Can you work these out from the model? Positions are in its coordinate system, mm. A direction names the side the tool comes from. Give positions to 0.01 mm unless a question says otherwise; leave off trailing zeros. Write each loop counter-clockwise with the first axis right and the second up, starting at its lowest first coordinate (ties: lowest second). Pieces come first, ordered by that corner, then holes. Notation, with made-up numbers: M 86,29.5 L 130,29.5 A10 ccw 130,35.5 Z; hole C -27,-25.5 d4. An arc over 180 degrees is marked long. Use CSV: the item, a comma, the result in double quotes. Start each with the question number.
from build123d import *

# Parameters (mm, degrees)
SKETCH_1_R               = 8
EXTRUDE_1_DEPTH          = 19.5
SKETCH_2_R               = 21
EXTRUDE_2_DEPTH          = 4
SKETCH_3_R               = 1.525
CUT_EXTRUDE_1_DEPTH      = 4
SKETCH_5_W               = 16
SKETCH_5_H               = 19.5
EXTRUDE_3_DEPTH          = 8
SKETCH_8_R               = 5
EXTRUDE_4_DEPTH          = 10
HOLE_WIZARD_G1_8_1_D     = 8.8
HOLE_WIZARD_G1_8_1_DEPTH = 11
HOLE_WIZARD_G1_8_1_TIP   = 2.643786724
CUT_EXTRUDE_4_REACH      = 35.5
SKETCH_9_R               = 2.025
FILLET_1_R               = 2
CHAMFER_1_SIZE           = 0.5


with BuildPart() as part:
    # 草图1 → 凸台-拉伸1 (new body)
    with BuildSketch(Plane(origin=(0, 0, 0), x_dir=(1, 0, 0), z_dir=(0, 1, 0))):
        Circle(SKETCH_1_R)
    extrude(amount=EXTRUDE_1_DEPTH)

    # 草图2 → 凸台-拉伸2 (add)
    with BuildSketch(Plane(origin=(0, 19.5, 0), x_dir=(1, 0, 0), z_dir=(0, 1, 0))):
        Circle(SKETCH_2_R)
    extrude(amount=EXTRUDE_2_DEPTH)

    # 草图3 → 切除-拉伸1 (cut)
    with BuildSketch(Plane.XZ.offset(-19.5)):
        with Locations((0, -13.5)):
            Circle(SKETCH_3_R)
        with Locations((-11.691342951, -6.75)):
            Circle(SKETCH_3_R)
        with Locations((-11.691342951, 6.75)):
            Circle(SKETCH_3_R)
        with Locations((0, 13.5)):
            Circle(SKETCH_3_R)
        with Locations((11.691342951, 6.75)):
            Circle(SKETCH_3_R)
        with Locations((11.691342951, -6.75)):
            Circle(SKETCH_3_R)
    extrude(amount=-CUT_EXTRUDE_1_DEPTH, mode=Mode.SUBTRACT)

    # 草图5 → 凸台-拉伸3 (add)
    with BuildSketch(Plane.XY):
        with Locations((0, 9.75)):
            Rectangle(SKETCH_5_W, SKETCH_5_H)
    extrude(amount=EXTRUDE_3_DEPTH)

    # 草图8 → 凸台-拉伸4 (add)
    with BuildSketch(Plane.XZ):
        Circle(SKETCH_8_R)
    extrude(amount=EXTRUDE_4_DEPTH)

    # G1/8 螺纹孔1
    with Locations(Plane(origin=(0, 9.75, 8), x_dir=(1, 0, 0), z_dir=(0, 0, 1))):
        with Locations((0, 0)):
            Hole(HOLE_WIZARD_G1_8_1_D / 2, depth=HOLE_WIZARD_G1_8_1_DEPTH)
            with Locations((0, 0, -(HOLE_WIZARD_G1_8_1_DEPTH + HOLE_WIZARD_G1_8_1_TIP / 2))):  # 118° drill point
                Cone(0, HOLE_WIZARD_G1_8_1_D / 2, HOLE_WIZARD_G1_8_1_TIP, mode=Mode.SUBTRACT)

    # 草图9 → 切除-拉伸4 (cut, up to next)
    with BuildSketch(Plane.XZ.offset(10), mode=Mode.PRIVATE) as cut_extrude_4_sk1:
        Circle(SKETCH_9_R)
    cut_extrude_4_tool1 = extrude(cut_extrude_4_sk1.sketch, amount=-CUT_EXTRUDE_4_REACH, mode=Mode.PRIVATE) & part.part
    add(cut_extrude_4_tool1.solids().sort_by_distance((0, -10, 0))[0], mode=Mode.SUBTRACT)

    # 圆角1
    fillet_1_edges = [part.edges().sort_by_distance(p)[0] for p in [
        (8, 9.75, 8),
        (-8, 9.75, 8),
    ]]
    fillet(fillet_1_edges, radius=FILLET_1_R)

    # 倒角1
    chamfer_1_edges = [part.edges().sort_by_distance(p)[0] for p in [
        (-21, 19.5, 0),
        (-21, 23.5, 0),
    ]]
    chamfer(chamfer_1_edges, length=CHAMFER_1_SIZE)


solid = part.part
(1) I want a section at A-A (y = 2). Write out the boundary of the cut face in (x, z) (3 decimals), and give its area (3 significant figures).
(2) Thinking about a two-plate mould opening in X: for faces 1 (the face through (9, 19.5, 0)), 2 (the face through (-2.365, 13.46, 2.423)), 3 (the face through (-8, 10, 3)), which applies, released by +X, released by -X, zero draft, split by the parting line, or undercut?
(3) I want a section at B-B (z = 6.75). State how many separate pieces and enclosed holes the cut face has, and give its area (3 significant figures).
(4) Which directions (+Z, -Z, +X, -X, +Y, -Y) give clear straight access to the entire face, cutting with the end or side of a thin tool? Please do faces 4 (the face through (0, 10, -8)), 5 (the face through (8, 10, 3)), 6 (the face through (-1.4, 14.2, 8)), 7 (the face through (-1.08, -4.93, -4.88)).
(5) Will these pins go through, and if not, where does the flat tip stop? pin 1 Ø5 at (y, z) = (0, -12.5) entering from -X; pin 2 Ø3 at (y, z) = (7, 2) entering from +X; pin 3 Ø6.5 at (y, z) = (6.5, 2) entering from -X; pin 4 Ø5 at (x, z) = (11.69, 6.75) entering from -Y.
(6) Please list where these lines run through material, in increasing order: L1, parallel to X at y = 20, z = -6; L2, parallel to Z at x = 0, y = -2 (3 decimals); L3, parallel to Z at x = 0, y = 2 (3 decimals). Write a range as [from, to].
Geometry results:
1,outline,"M -8,0 A8 ccw 8,0 L 8,6 A2 ccw 6,8 L -6,8 A2 ccw -8,6 Z; hole C 0,0 d4.05"
1,area,"214 mm2"
2,face 1,"zero draft"
2,face 2,"undercut"
2,face 3,"released by -X"
3,separate pieces,"3"
3,enclosed holes,"1"
3,area,"380 mm2"
4,face 4,"-Z, -Y"
4,face 5,"+Z, -Z, +X, -Y"
4,face 6,"+Z, +X, -X, -Y"
4,face 7,"-Y"
5,pin 1,"passes through"
5,pin 2,"stops at x = 8"
5,pin 3,"stops at x = -8"
5,pin 4,"stops at y = 19.5"
6,L1,"x = [-20.12, -13.02], [-10.36, 10.36], [13.02, 20.12]"
6,L2,"z = [-5, -2.025], [2.025, 5]"
6,L3,"z = [-8, -2.025], [2.025, 8]"
